Here's how the part is built. I have some questions about the finished solid (model axes, mm). A direction names the side the tool comes from. Coordinates: 2 decimals unless noted, no trailing zeros. Write each loop counter-clockwise with the first axis right and the second up, starting at its lowest first coordinate (ties: lowest second). Pieces come first, ordered by that corner, then holes. Notation, with made-up numbers: M 73,70.5 L 104,70.5 A23 cw 104,90.5 Z; hole C 5.5,9.25 d10. An arc over 180 degrees is marked long. Use a Markdown table: item, result.
```python
from build123d import *

# Parameters (mm, degrees)
BOSS_EXTRUDE1_DEPTH = 3.175


with BuildPart() as part:
    # Sketch1 → Boss-Extrude1 (new body)
    with BuildSketch(Plane(origin=(0, 0, 0), x_dir=(0, 0, -1), z_dir=(1, 0, 0))):
        Polygon((0, 110.49), (3.175, 110.49), (3.175, 91.44), (0, 91.44), (0, 72.39), (3.175, 72.39), (3.175, 53.34), (0, 53.34), (0, 34.29), (3.175, 34.29), (3.175, 15.24), (0, 15.24), (0, 0), (-63.5, 0), (-63.5, 15.24), (-66.675, 15.24), (-66.675, 34.29), (-63.5, 34.29), (-63.5, 53.34), (-66.675, 53.34), (-66.675, 72.39), (-63.5, 72.39), (-63.5, 91.44), (-66.675, 91.44), (-66.675, 110.49), (-63.5, 110.49), (-63.5, 133.35), (0, 133.35), align=None)
    extrude(amount=BOSS_EXTRUDE1_DEPTH)


solid = part.part
```
1. Which directions (+Z, -Z, +X, -X, +Y, -Y) give clear straight access to the entire face, cutting with the end or side of a thin tool? Please do faces 1 (the face through (2, 91.44, -2)), 2 (the face through (2, 72.39, 65)), 3 (the face through (2, 15.24, -2)).
Answers follow:
| item | result |
|---|---|
| face 1 | -Z, +X, -X |
| face 2 | +Z, +X, -X |
| face 3 | -Z, +X, -X, -Y |
2. I need wall thicknesses on probe 1 along Z at (x, y) = (0.8, 10). Which ranges of the line are inside material? Lowest first, please.
Answers follow:
| item | result |
|---|---|
| probe 1 | z = 0 to 63.5 |
3. Suppose I cut it at B-B on y = 36. Write out the boundary of the cut face in (x, z) (3 decimals), and give its area (3 significant figures).
Answers follow:
| item | result |
|---|---|
| outline | M 0,0 L 3.175,0 L 3.175,63.5 L 0,63.5 Z |
| area | 202 mm2 |
4. Will these pins go through, and if not, where does the flat tip stop? pin 1 Ø1.6 at (x, z) = (1.5, 65) entering from +Y; pin 2 Ø1 at (x, y) = (2.5, 47) entering from -Z; pin 3 Ø1 at (x, z) = (1.5, 64.5) entering from -Y.
Answers follow:
| item | result |
|---|---|
| pin 1 | stops at y = 110.49 |
| pin 2 | stops at z = 0 |
| pin 3 | stops at y = 15.24 |
5. Suppose I cut it at A-A on x = 1.35. Write out the boundary of the cut face in (y, z) (3 decimals).
Answers follow:
| item | result |
|---|---|
| outline | M 0,0 L 15.24,0 L 15.24,-3.175 L 34.29,-3.175 L 34.29,0 L 53.34,0 L 53.34,-3.175 L 72.39,-3.175 L 72.39,0 L 91.44,0 L 91.44,-3.175 L 110.49,-3.175 L 110.49,0 L 133.35,0 L 133.35,63.5 L 110.49,63.5 L 110.49,66.675 L 91.44,66.675 L 91.44,63.5 L 72.39,63.5 L 72.39,66.675 L 53.34,66.675 L 53.34,63.5 L 34.29,63.5 L 34.29,66.675 L 15.24,66.675 L 15.24,63.5 L 0,63.5 Z |
6. We'd pull the mould along Y, two halves only. Please class faces 4 (the face through (2, 101, -3.175)), 5 (the face through (2, 53.34, 65)), 6 (the face through (2, 82, 0)), 7 (the face through (2, 15.24, 65)): +Y half, -Y half, draft (parallel to the pull), parting line (faces both ways), or undercut.
Answers follow:
| item | result |
|---|---|
| face 4 | draft |
| face 5 | undercut |
| face 6 | undercut |
| face 7 | -Y half |
